from build123d import *

# Parameters (mm, degrees)
SKETCH1_R                = 13
BOSS_EXTRUDE1_DEPTH      = 4
CHAMFER1_SIZE            = 30
M3_CLEARANCE_HOLE1_D     = 3.2
M3_CLEARANCE_HOLE1_DEPTH = 8
M3_CLEARANCE_HOLE1_TIP   = 0.96137699
FILLET1_R                = 5
M5_CLEARANCE_HOLE1_D     = 5.5
M5_CLEARANCE_HOLE1_DEPTH = 8
M5_CLEARANCE_HOLE1_TIP   = 1.652366702


with BuildPart() as part:
    # Sketch1 → Boss-Extrude1 (new body)
    with BuildSketch(Plane(origin=(0, 0, 0), x_dir=(1, 0, 0), z_dir=(0, 1, 0))):
        Polygon((-69, -60), (-69, 43), (69, 43), (69, -60), (39, -60), (39, 0), (-39, 0), (-39, -60), align=None)
        with Locations(Location((0, 20, 0), (0, 0, 270))):
            Circle(SKETCH1_R, mode=Mode.SUBTRACT)
    extrude(amount=BOSS_EXTRUDE1_DEPTH)

    # Chamfer1
    chamfer1_edges = [part.edges().sort_by_distance(p)[0] for p in [
        (-69, 2, -43),
        (69, 2, -43),
    ]]
    chamfer(chamfer1_edges, length=CHAMFER1_SIZE)

    # M3 Clearance Hole1
    with Locations(Plane(origin=(0, 4, 0), x_dir=(1, 0, 0), z_dir=(0, 1, 0))):
        with Locations((-15.5, 35.5), (-15.5, 4.5), (15.5, 4.5), (15.5, 35.5)):
            Hole(M3_CLEARANCE_HOLE1_D / 2, depth=M3_CLEARANCE_HOLE1_DEPTH)
            with Locations((0, 0, -(M3_CLEARANCE_HOLE1_DEPTH + M3_CLEARANCE_HOLE1_TIP / 2))):  # 118° drill point
                Cone(0, M3_CLEARANCE_HOLE1_D / 2, M3_CLEARANCE_HOLE1_TIP, mode=Mode.SUBTRACT)

    # Fillet1
    fillet1_edges = [part.edges().sort_by_distance(p)[0] for p in [
        (-69, 2, 60),
        (69, 2, 60),
        (-69, 2, -13),
        (39, 2, -43),
        (-39, 2, -43),
        (69, 2, -13),
    ]]
    fillet(fillet1_edges, radius=FILLET1_R)

    # M5 Clearance Hole1
    with Locations(Plane(origin=(0, 4, 0), x_dir=(1, 0, 0), z_dir=(0, 1, 0))):
        with Locations((-54, -47), (-54, -17), (54, -17), (54, -47)):
            Hole(M5_CLEARANCE_HOLE1_D / 2, depth=M5_CLEARANCE_HOLE1_DEPTH)
            with Locations((0, 0, -(M5_CLEARANCE_HOLE1_DEPTH + M5_CLEARANCE_HOLE1_TIP / 2))):  # 118° drill point
                Cone(0, M5_CLEARANCE_HOLE1_D / 2, M5_CLEARANCE_HOLE1_TIP, mode=Mode.SUBTRACT)


solid = part.part
Read the model definition and answer for the solid it produces. Units are mm, in the model's axes. A direction names the side the tool comes from. Give positions to 0.01 mm unless a question says otherwise; leave off trailing zeros. Write each loop counter-clockwise with the first axis right and the second up, starting at its lowest first coordinate (ties: lowest second). Pieces come first, ordered by that corner, then holes. Notation, with made-up numbers: (55.25, 38.25) - (95.25, 38.25) arc R21 cw to (95.25, 47.25) - close; hole circle Ø7 at (73, -24.5). An arc over 180 degrees is marked (long way). Use CSV: the item, a comma, the result in double quotes. Start each with the question number.
Item 1: The part is cut by section B-B, the plane x = 0. Give the vertices of the cut face in (y, z).
Item 2: The part is cut by section A-A, the plane z = -4.5. Give the vertices of the cut face in (x, y).
Item 3: The mould has two halves that part along X. Classify faces 1 (the cylindrical face through (17.1, 1.97, -4.57)), 2 (the cylindrical face through (68, 2, 58)), 3 (the flat face through (-54, 2, -28)): pulls with the +X half, pulls with the -X half, needs draft (parallel to the pull), parting line crosses it, or undercut.
Item 4: For faces 4 (the flat face through (39, 2, 30)), 5 (the cylindrical face through (68.61, 2.03, -12.87)), determine the directions among +Z, -Z, +X, -X, +Y, -Y from which every point of the face is accessible in a straight line to the end or side of a thin tool.
Item 5: The part is cut by section C-C, the plane y = 2.15. Count the separate pieces of the cut face and the enclosed holes in it, and give its area (3 significant figures).
Item 6: Flat-ended cylindrical pins translate along their axes: P1, Ø2.5, axis at x = -15.5, z = -35.5, coming from the +Y side; P2, Ø7, axis at x = 54, z = 47, coming from the +Y side; P3, Ø2, axis at x = 10.5, y = 1.5, coming from the +Z side. Find the tip coordinate at first contact, or state that the pin passes through.
Item 7: Consider line 1 (Z direction, x = -15.5, y = 2.95); line 2 (X direction, y = 1.85, z = 47); line 3 (X direction, y = 0.3, z = 21). Determine where each line is inside the solid, lowest interval first.
Item 8: The part is cut by section D-D, the plane x = 15.5. Give the vertices of the cut face in (y, z).
Taken from the geometry:
1,outline,"(0, -43) - (4, -43) - (4, -33) - (0, -33) - close; (0, -7) - (4, -7) - (4, 0) - (0, 0) - close"
2,outline,"(-69, 0) - (-17.1, 0) - (-17.1, 4) - (-69, 4) - close; (-13.9, 0) - (13.9, 0) - (13.9, 4) - (-13.9, 4) - close; (17.1, 0) - (69, 0) - (69, 4) - (17.1, 4) - close"
3,face 1,"undercut"
3,face 2,"pulls with the +X half"
3,face 3,"pulls with the -X half"
4,face 4,"+Z, +Y, -Y"
4,face 5,"-Z, +X, +Y, -Y"
5,separate pieces,"1"
5,enclosed holes,"9"
5,area,"7,960 mm2"
6,P1,"through"
6,P2,"y = 4"
6,P3,"z = 0"
7,line 1,"-43 to -37.1, -33.9 to -6.1, -2.9 to 0"
7,line 2,"-69 to -56.75, -51.25 to -39, 39 to 51.25, 56.75 to 69"
7,line 3,"-69 to -39, 39 to 69"
8,outline,"(0, -43) - (4, -43) - (4, -37.1) - (0, -37.1) - close; (0, -33.9) - (4, -33.9) - (4, -6.1) - (0, -6.1) - close; (0, -2.9) - (4, -2.9) - (4, 0) - (0, 0) - close"
